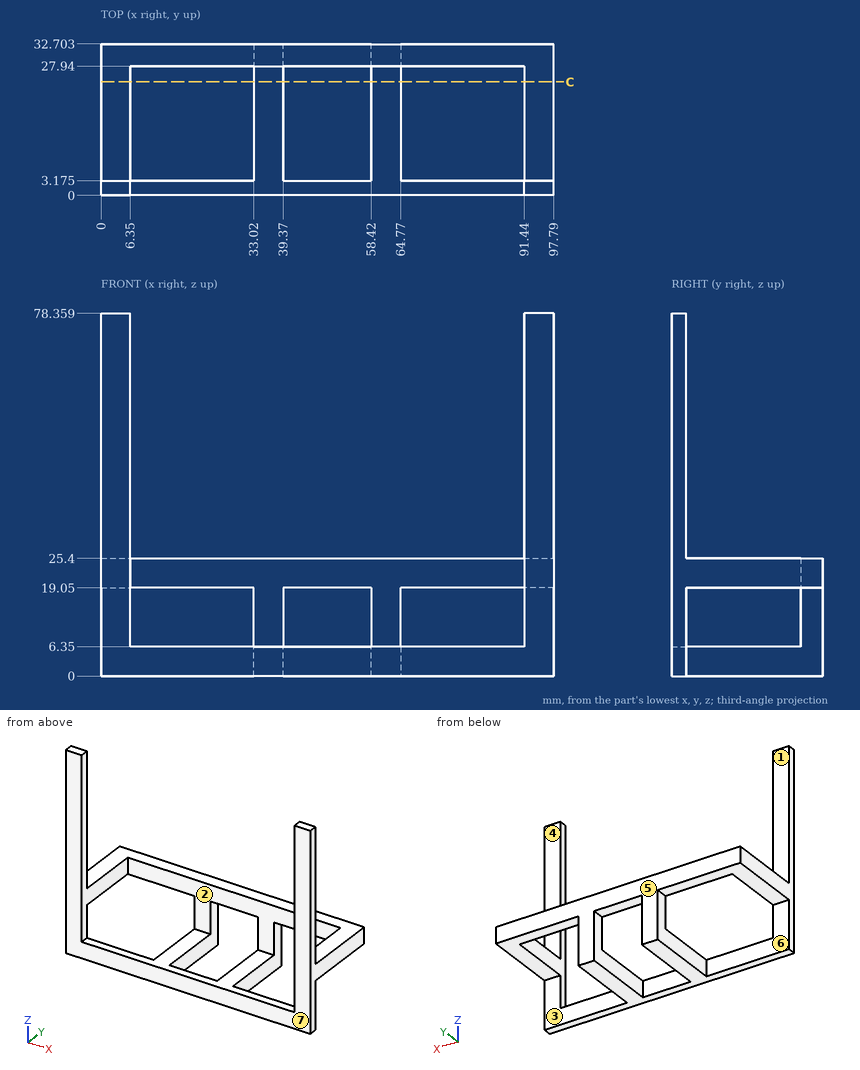
The figure shows three views and two pictorial views of one solid part (mm, origin at its lowest corner). Answer the questions. A direction names the side the tool comes from. Give positions to 0.01 mm unless a question says otherwise; leave off trailing zeros. Order: outer loops, then holes, each group sorted by start corner. A loop starts at its lowest first (then second) coordinate and runs counter-clockwise, first axis right, second up. Notation, with made-up numbers: (12.25, -18) -> (65.25, -18) arc R24 ccw to (65.25, -6) -> close; hole circle Ø10 at (56.5, -5). An arc over 180 degrees is marked (long way). Answer as a JSON object with one key per item and string values. Group by question number.
Item 1: Determine the mould class of the marked faces 1 and 2 for opening direction X: pulls with the +X half, pulls with the -X half, needs draft (parallel to the pull), parting line crosses it, or undercut.
Item 2: A tool of negligible diameter and unlimited length cuts with its end or side. For the marked faces 3, 4, 5, 6 and 7, from which of +Z, -Z, +X, -X, +Y, -Y can it reach the whole face along a straight path? Write none if from no direction.
Item 3: The part is cut by section C-C on y = 24.5. Write down the section's boundary in (x, z).
Item 4: Consider L1, parallel to X at y = 30, z = 11; L2, parallel to X at y = 2.5, z = 13; L3, parallel to Z at x = 24, y = 29.5. Determine where each line is inside the solid, lowest interval first. Write a range as from..to.
Item 5: Flat-ended cylindrical pins translate along their axes: pin 1 (15 mm diameter, centred on x = 24, y = 12.5, fed in from -Z); pin 2 (3 mm diameter, centred on x = 2.5, z = 49, fed in from +Y) (1 decimal); pin 3 (15 mm diameter, centred on y = 19.5, z = 6, fed in from +X); pin 4 (14 mm diameter, centred on y = 14, z = 31, fed in from +X). Find the tip coordinate at first contact, or state that the pin passes through.
Result set:
{
 "1": {"face 1": "needs draft", "face 2": "undercut"},
 "2": {"face 3": "-Z, +X, +Y", "face 4": "+Z, +X, -X, +Y", "face 5": "+Z, -Z, +X, -X, +Y", "face 6": "-Z, -X, +Y", "face 7": "+Z, -Z, +X, -X, -Y"},
 "3": {"outline": "(0, 19.05) -> (6.35, 19.05) -> (6.35, 25.4) -> (0, 25.4) -> close; (33.02, 0) -> (39.37, 0) -> (39.37, 6.35) -> (33.02, 6.35) -> close; (58.42, 0) -> (64.77, 0) -> (64.77, 6.35) -> (58.42, 6.35) -> close; (91.44, 19.05) -> (97.79, 19.05) -> (97.79, 25.4) -> (91.44, 25.4) -> close"},
 "4": {"L1": "33.02..39.37, 58.42..64.77", "L2": "0..6.35, 91.44..97.79", "L3": "19.05..25.4"},
 "5": {"pin 1": "through", "pin 2": "y = 3.2", "pin 3": "x = 64.77", "pin 4": "x = 97.79"}
}
